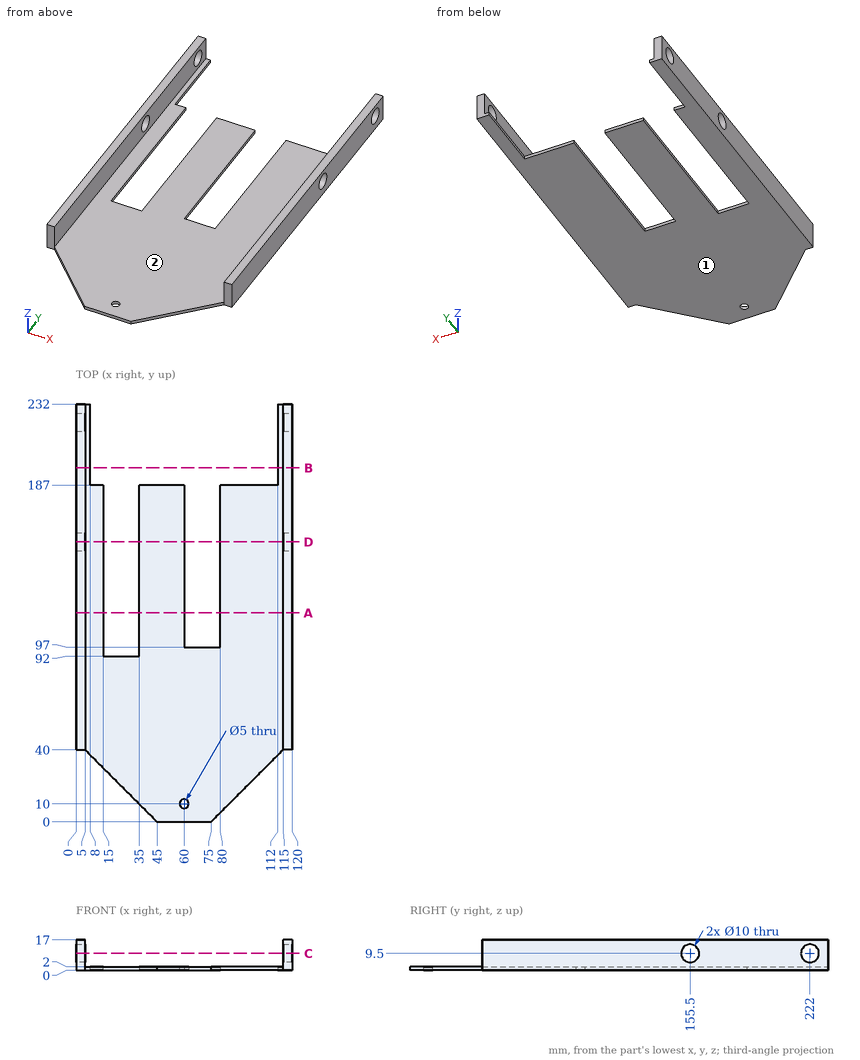
Print and shaded views of the part. All mm, measured from the part's lowest x, y and z. A direction names the side the tool comes from. Coordinates: 2 decimals unless noted, no trailing zeros. Loops run counter-clockwise (first coordinate to the right, second up) from the corner with the lowest first, then second, coordinate; pieces in that order, holes last. Notation, with made-up numbers: (-21.75, -28.75) -> (35.25, -28.75) arc R30 ccw to (35.25, 1.25) -> close; hole circle Ø3 at (77, 5.5). An arc over 180 degrees is marked (long way). Use a Markdown table: item, result. Add a question column.
Item 1: Band-saw the part on C-C on z = 9.5. Write the cut outline in (x, y), plus the area to 3 significant figures.
Item 2: Band-saw the part on A-A on y = 116. Write the cut outline in (x, z).
Item 3: Probe probe 1 along Y at (x, z) = (3.25, 9.5); probe 2 along X at (y, z) = (132.5, 1.75); probe 3 along X at (y, z) = (173, 6.25). List the from-to ranges inside material, lowest first.
Item 4: Flat gauge pins, fed straight in: P1, Ø1.5, axis at x = 69, y = 36.5, coming from the +Z side; P2, Ø1.6, axis at x = 20.5, z = 1, coming from the +Y side; P3, Ø1.5, axis at x = 106, y = 187.5, coming from the -Z side; P4, Ø2.5, axis at x = 2, z = 7, coming from the -Y side. Where does each tip first touch, or does it go through?
Item 5: Band-saw the part on B-B on y = 196.5. Write the cut outline in (x, z).
Item 6: Which spindle directions (+Z, -Z, +X, -X, +Y, -Y) get a long thin tool onto all of the face, cutting with end or side? Do the marked faces 1 and 2. Say none if no direction does.
Item 7: Band-saw the part on D-D on y = 155.5. Write the cut outline in (x, z).
Geometry says:
| question | item | result |
|---|---|---|
| 1 | outline | (0, 40) -> (5, 40) -> (5, 150.5) -> (0, 150.5) -> close; (0, 160.5) -> (5, 160.5) -> (5, 217) -> (0, 217) -> close; (0, 227) -> (5, 227) -> (5, 232) -> (0, 232) -> close; (115, 40) -> (120, 40) -> (120, 150.5) -> (115, 150.5) -> close; (115, 160.5) -> (120, 160.5) -> (120, 217) -> (115, 217) -> close; (115, 227) -> (120, 227) -> (120, 232) -> (115, 232) -> close |
| 1 | area | 1,720 mm² |
| 2 | outline | (0, 0) -> (15, 0) -> (15, 2) -> (5, 2) -> (5, 17) -> (0, 17) -> close; (35, 0) -> (60, 0) -> (60, 2) -> (35, 2) -> close; (80, 0) -> (120, 0) -> (120, 17) -> (115, 17) -> (115, 2) -> (80, 2) -> close |
| 3 | probe 1 | 40 to 150.5, 160.5 to 217, 227 to 232 |
| 3 | probe 2 | 0 to 15, 35 to 60, 80 to 120 |
| 3 | probe 3 | 0 to 5, 115 to 120 |
| 4 | P1 | z = 2 |
| 4 | P2 | y = 92 |
| 4 | P3 | z = 0 |
| 4 | P4 | y = 40 |
| 5 | outline | (0, 0) -> (8, 0) -> (8, 2) -> (5, 2) -> (5, 17) -> (0, 17) -> close; (112, 0) -> (120, 0) -> (120, 17) -> (115, 17) -> (115, 2) -> (112, 2) -> close |
| 6 | face 1 | -Z, +X, -X, +Y, -Y |
| 6 | face 2 | +Z, +Y, -Y |
| 7 | outline | (0, 0) -> (15, 0) -> (15, 2) -> (5, 2) -> (5, 4.5) -> (0, 4.5) -> close; (0, 14.5) -> (5, 14.5) -> (5, 17) -> (0, 17) -> close; (35, 0) -> (60, 0) -> (60, 2) -> (35, 2) -> close; (80, 0) -> (120, 0) -> (120, 4.5) -> (115, 4.5) -> (115, 2) -> (80, 2) -> close; (115, 14.5) -> (120, 14.5) -> (120, 17) -> (115, 17) -> close |
